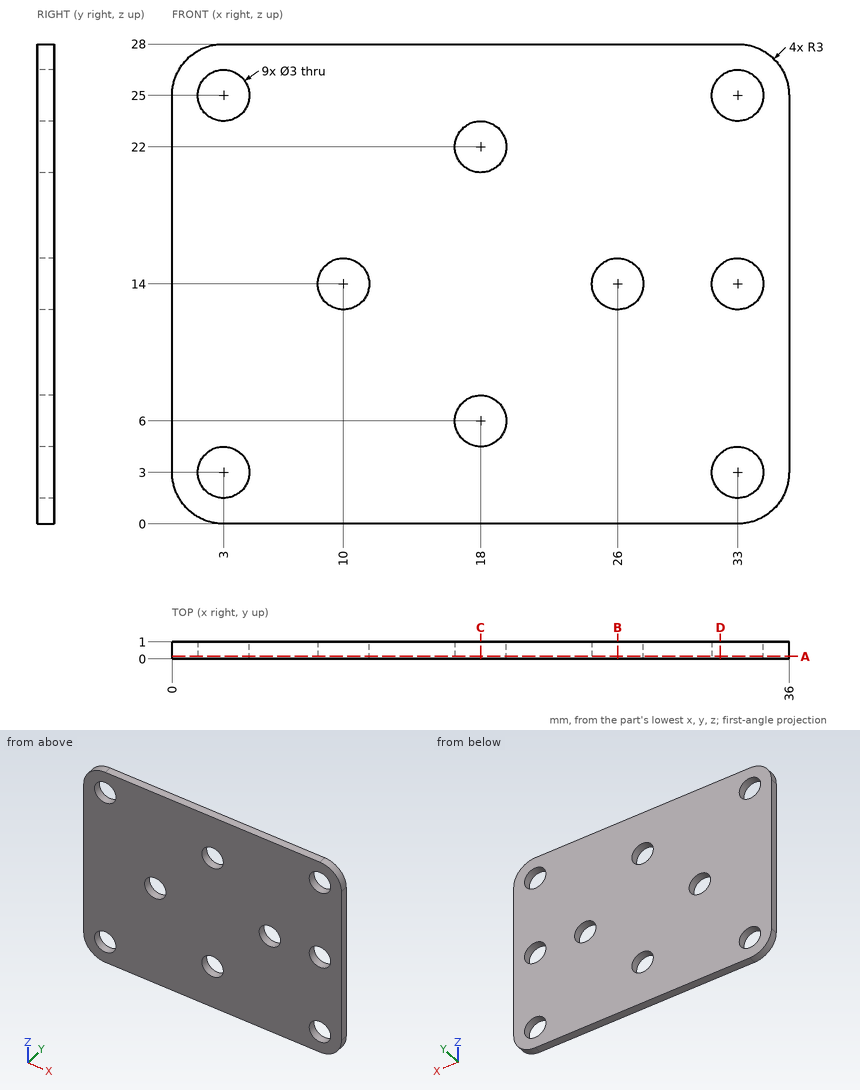
Job drawing, mm, ordinate dimensions from the low corner. One solid piece. Give positions to 0.01 mm unless a question says otherwise; leave off trailing zeros. Loops run counter-clockwise (first coordinate to the right, second up) from the corner with the lowest first, then second, coordinate; pieces in that order, holes last. Notation, with made-up numbers: M 73.5,64 L 104.5,64 A27 cw 104.5,88 Z; hole C 72,67 d3. An arc over 180 degrees is marked long. Return JSON: item names as keys, results as strings.
1) Saw through at B-B, the plane x = 26. List the corners of the cut face in (y, z).
Calculated:
{"outline": "M 0,0 L 1,0 L 1,12.5 L 0,12.5 Z; M 0,15.5 L 1,15.5 L 1,28 L 0,28 Z"}
2) Drill centre lines: line 1 (X direction, y = 0.5, z = 3); line 2 (Z direction, x = 18, y = 0.35); line 3 (Z direction, x = 10, y = 0.45). Where is each one in solid material? Low to high.
Calculated:
{"line 1": "x = 0 to 1.5, 4.5 to 31.5, 34.5 to 36", "line 2": "z = 0 to 4.5, 7.5 to 20.5, 23.5 to 28", "line 3": "z = 0 to 12.5, 15.5 to 28"}
3) Saw through at C-C, the plane x = 18. List the corners of the cut face in (y, z).
Calculated:
{"outline": "M 0,0 L 1,0 L 1,4.5 L 0,4.5 Z; M 0,7.5 L 1,7.5 L 1,20.5 L 0,20.5 Z; M 0,23.5 L 1,23.5 L 1,28 L 0,28 Z"}
4) Saw through at A-A, the plane y = 0.15. Count the separate pieces of the cut face and the enclosed holes in it, then the cut area to 3 significant figures.
Calculated:
{"separate pieces": "1", "enclosed holes": "9", "area": "937 mm2"}
5) Saw through at D-D, the plane x = 32. List the corners of the cut face in (y, z).
Calculated:
{"outline": "M 0,0 L 1,0 L 1,1.88 L 0,1.88 Z; M 0,4.12 L 1,4.12 L 1,12.88 L 0,12.88 Z; M 0,15.12 L 1,15.12 L 1,23.88 L 0,23.88 Z; M 0,26.12 L 1,26.12 L 1,28 L 0,28 Z"}
